from build123d import *

# Parameters (mm, degrees)
F0_R          = 2.5
F4_DEPTH      = 2.5010001
F4_DEPTH_BACK = 2.5010001
F5_SIZE       = 0.388


with BuildPart() as f2:
    # F2: sweep along a path in F1
    with BuildLine(Plane.XZ) as f2_path:
        Line((0, 0), (0, 30))
        ThreePointArc((0, 30), (-14.5, 44.5), (-29, 30))
        Line((-29, 30), (-29, 10))
    # F0 (on Top) → F2 (sweep)
    with BuildSketch(Plane.XY):
        Circle(F0_R)
    sweep(path=f2_path.line)

    # F3 (on Front) → F4 (cut, two sides)
    with BuildSketch(Plane.XZ) as f4_sk:
        Polygon((-29, 13.5), (-29, 12.3), (-24.9849649455, 12.3), (-24.9849649455, 19.23406431), align=None)
        Polygon((-4.0150350545, 19.23406431), (-4.0150350545, 12.3), (0, 12.3), (0, 13.5), align=None)
    extrude(amount=-F4_DEPTH, mode=Mode.SUBTRACT)
    extrude(f4_sk.sketch, amount=F4_DEPTH_BACK, mode=Mode.SUBTRACT)

    # F5
    f5_edges = [f2.edges().sort_by_distance(p)[0] for p in [
        (-26.5, 0, 10),
        (-2.5, 0, 0),
    ]]
    chamfer(f5_edges, length=F5_SIZE)


solid = f2.part
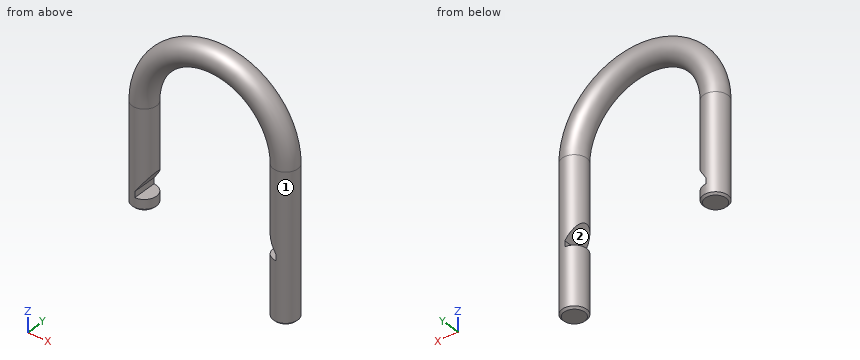
Design review of the part built by this model. Coordinates are the model's own, in mm. Face numbers are marked on the shaded views. A direction names the side the tool comes from. Give positions to 0.01 mm unless a question says otherwise; leave off trailing zeros. Loops run counter-clockwise (first coordinate to the right, second up) from the corner with the lowest first, then second, coordinate; pieces in that order, holes last. Notation, with made-up numbers: (85.5, 19.25) - (122.5, 19.25) arc R19 ccw to (122.5, 28.25) - close; hole circle Ø4 at (1, 13). An arc over 180 degrees is marked (long way). Use CSV: the item, a comma, the result in double quotes. Start each with the question number.
1. Insertion check: P1, Ø1, axis at y = 1.5, z = 10.5, coming from the +X side; P2, Ø2, axis at x = -28, y = 0, coming from the -Z side; P3, Ø1.2, axis at x = -27, y = -0.5, coming from the +Z side. Each pin has a flat end and moves straight along its axis. Give the tip position at first contact, or say it passes through.
2. Wall thickness on L1, parallel to X at y = 0.1, z = 19.5; L2, parallel to Y at x = -16.5, z = 43; L3, parallel to X at y = 2.25, z = 11: over which ranges is each line inside the solid? List them lowest first.
3. Add section A-A (z = 25). State the section outline as (x, y) points, plus the area to 3 significant figures.
4. Add section B-B (y = 0). State the section outline as (x, z) points, plus the area to 3 significant figures.
5. Machinability: for the marked faces 1 and 2, which of the approach directions +Z, -Z, +X, -X, +Y, -Y give a long, thin tool a straight path to every point of the face, cutting with its end or side? Answer none if there is none.
6. Add section C-C (z = 9). State the section outline as (x, y) points.
Results found:
1,P1,"stops at x = 2.29"
1,P2,"stops at z = 10"
1,P3,"stops at z = 42.09"
2,L1,"x = -31.5 to -26.5, -2.5 to 2.5"
2,L2,"y = -2.11 to 2.11"
2,L3,"x = -30.09 to -27.91, -1.09 to 1.09"
3,outline,"circle Ø5 at (-29, 0); circle Ø5 at (0, 0)"
3,area,"39.3 mm²"
4,outline,"(-31.5, 10.39) - (-31.11, 10) - (-26.89, 10) - (-26.5, 10.39) - (-26.5, 12.3) - (-29, 12.3) - (-29, 13.5) - (-26.5, 17.07) - (-26.5, 30) arc R12 cw to (-2.5, 30) - (-2.5, 17.07) - (0, 13.5) - (0, 12.3) - (-2.5, 12.3) - (-2.5, 0.39) - (-2.11, 0) - (2.11, 0) - (2.5, 0.39) - (2.5, 30) arc R17 ccw to (-31.5, 30) - close"
4,area,"463 mm²"
5,face 1,"-Z"
5,face 2,"+Y, -Y"
6,outline,"circle Ø5 at (0, 0)"
